Check sheet for the modelled part. Datum: model origin and axes. Units: mm. Face numbers are marked on the shaded views. A direction names the side the tool comes from. Round coordinates to 2 decimals unless told otherwise and drop trailing zeros. Loops run counter-clockwise (first coordinate to the right, second up) from the corner with the lowest first, then second, coordinate; pieces in that order, holes last. Notation, with made-up numbers: (74.5, -15.5) - (89.5, -15.5) arc R24 cw to (89.5, 8.5) - close; hole circle Ø3 at (-5, 23). An arc over 180 degrees is marked (long way). Put each result on its own line as item: value. Start each with the question number.
Item 1: Section check D-D, the plane y = 74.5. Record the cut outline in (x, z), and give its area (3 significant figures).
Item 2: Gauge pin test, flat ends, axial feed: pin 1 Ø1.5 at (x, z) = (24.5, -60) entering from +Y; pin 2 Ø12.5 at (x, y) = (103.5, 4.5) entering from -Z; pin 3 Ø12 at (x, z) = (109.5, -23.5) entering from +Y. Record the tip position at first contact, or that the pin passes through.
Item 3: Tool access check on the marked faces 1 and 2. Record the directions out of +Z, -Z, +X, -X, +Y, -Y that give a thin tool (end or side, any length) a straight path to the whole face; none if there is none.
Item 4: Material ranges on line 1 along Z through (x, y) = (133.5, 4.5); line 2 along X through (y, z) = (48, -37); line 3 along Y through (x, z) = (143.5, -25), recorded low to high.
Item 5: Section check B-B, the plane x = 22.5. Record the cut outline in (y, z), and give its area (3 significant figures).
Item 6: Section check C-C, the plane z = -63.5. Record the cut outline in (x, y).
Item 7: Section check A-A, the plane x = 89. Record the cut outline in (y, z).
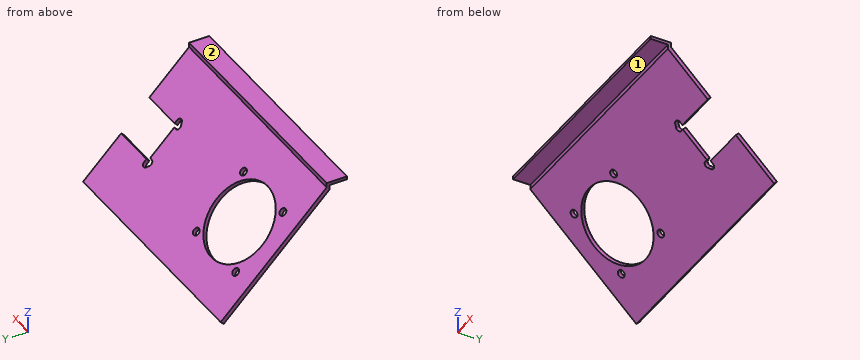
from build123d import *

# Parameters (mm, degrees)
BOSS_EXTRUDE1_DEPTH = 160
BOSS_EXTRUDE2_DEPTH = 160
SKETCH4_W           = 31.25
SKETCH4_H           = 14
SKETCH4_H_2         = 12.5
CUT_EXTRUDE1_DEPTH  = 10
CUT_EXTRUDE2_DEPTH  = 10
SKETCH6_R           = 26.5
CUT_EXTRUDE3_DEPTH  = 10
SKETCH7_R           = 2.5
CUT_EXTRUDE4_DEPTH  = 10


with BuildPart() as part:
    # Sketch1 → Boss-Extrude1 (new body)
    with BuildSketch(Plane(origin=(0, 0, 0), x_dir=(0, 0, -1), z_dir=(1, 0, 0))):
        Polygon((0, 0), (0, 11.5), (3, 11.5), (3, 13.5), (-2, 13.5), (-2, 0), align=None)
    extrude(amount=BOSS_EXTRUDE1_DEPTH)

    # Sketch2 → Boss-Extrude2 (add)
    with BuildSketch(Plane(origin=(0, 0, 0), x_dir=(0, 0, -1), z_dir=(1, 0, 0))):
        Polygon((3, 13.5), (3, 11.5), (24.213203436, 32.713203436), (73.710678119, 82.210678119), (71.710678119, 84.210678119), (22.213203436, 34.713203436), (1, 13.5), align=None)
    extrude(amount=BOSS_EXTRUDE2_DEPTH)

    # Sketch4 → Cut-Extrude1 (cut)
    with BuildSketch(Plane(origin=(0, 6.25, 6.25), x_dir=(1, 0, 0), z_dir=(0, 0.7071067811865477, 0.7071067811865475))):
        with Locations((144.375, 67.253048327)):
            Rectangle(SKETCH4_W, SKETCH4_H)
        with Locations((144.375, 54.003048327)):
            Rectangle(SKETCH4_W, SKETCH4_H_2)
    extrude(amount=-CUT_EXTRUDE1_DEPTH, mode=Mode.SUBTRACT)

    # Sketch5 → Cut-Extrude2 (cut)
    with BuildSketch(Plane(origin=(0, 6.25, 6.25), x_dir=(1, 0, 0), z_dir=(0, 0.7071067811865477, 0.7071067811865475))):
        with BuildLine():
            Line((128.75, 74.253048327), (130.644024073, 74.253048327))
            Line((130.644024073, 74.253048327), (130.644024073, 76.548206166))
            ThreePointArc((130.644024073, 76.548206166), (129.12196275, 78.639811919), (126.663600689, 77.834863927))
            Line((126.663600689, 77.834863927), (125.199975137, 75.807473041))
            ThreePointArc((125.199975137, 75.807473041), (125.025166605, 73.519904499), (126.982233047, 72.322649807))
            Line((126.982233047, 72.322649807), (128.75, 72.322649807))
            Line((128.75, 72.322649807), (128.75, 74.253048327))
        make_face()
        with BuildLine():
            Line((128.75, 49.683446848), (126.982233047, 49.683446848))
            ThreePointArc((126.982233047, 49.683446848), (125.025166605, 48.486192156), (125.199975137, 46.198623614))
            Line((125.199975137, 46.198623614), (126.663600689, 44.171232728))
            ThreePointArc((126.663600689, 44.171232728), (129.12196275, 43.366284735), (130.644024073, 45.457890488))
            Line((130.644024073, 45.457890488), (130.644024073, 47.753048327))
            Line((130.644024073, 47.753048327), (128.75, 47.753048327))
            Line((128.75, 47.753048327), (128.75, 49.683446848))
        make_face()
    extrude(amount=-CUT_EXTRUDE2_DEPTH, mode=Mode.SUBTRACT)

    # Sketch6 → Cut-Extrude3 (cut)
    with BuildSketch(Plane(origin=(0, 6.25, 6.25), x_dir=(1, 0, 0), z_dir=(0, 0.7071067811865477, 0.7071067811865475))):
        with Locations(Location((38.75, 61.003048327, 0), (0, 0, 270))):
            Circle(SKETCH6_R)
    extrude(amount=-CUT_EXTRUDE3_DEPTH, mode=Mode.SUBTRACT)

    # Sketch7 → Cut-Extrude4 (cut)
    with BuildSketch(Plane(origin=(0, 6.25, 6.25), x_dir=(1, 0, 0), z_dir=(0, 0.7071067811865477, 0.7071067811865475))):
        with Locations(Location((15.82638188, 83.269496377, 0), (0, 0, 270))):
            Circle(SKETCH7_R)
        with Locations(Location((15.82638188, 38.736600277, 0), (0, 0, 270))):
            Circle(SKETCH7_R)
        with Locations(Location((61.67361812, 38.736600277, 0), (0, 0, 270))):
            Circle(SKETCH7_R)
        with Locations(Location((61.67361812, 83.269496377, 0), (0, 0, 270))):
            Circle(SKETCH7_R)
    extrude(amount=-CUT_EXTRUDE4_DEPTH, mode=Mode.SUBTRACT)


solid = part.part
Check result:
1. outline: (0, -66) - (160, -66) - (160, -62) - (0, -62) - close
1. area: 640 mm²
2. pin 1: y = 73.25
2. pin 2: z = 0
2. pin 3: y = 42
3. face 1: -Z, +X, -X, -Y
3. face 2: +Z, +X, -X, +Y, -Y
4. line 1: 0 to 2
4. line 2: 0 to 12.27, 65.23 to 128.75
4. line 3: 33.5 to 37.5
5. outline: (0, 0) - (11.5, 0) - (11.5, -3) - (32.58, -24.08) - (34.58, -22.08) - (13.5, -1) - (13.5, 2) - (0, 2) - close; (62.19, -53.69) - (82.21, -73.71) - (84.21, -71.71) - (64.19, -51.69) - close
5. area: 195 mm²
6. outline: (0, 72) - (160, 72) - (160, 76) - (0, 76) - close
7. outline: (0, 0) - (11.5, 0) - (11.5, -3) - (82.21, -73.71) - (84.21, -71.71) - (13.5, -1) - (13.5, 2) - (0, 2) - close
